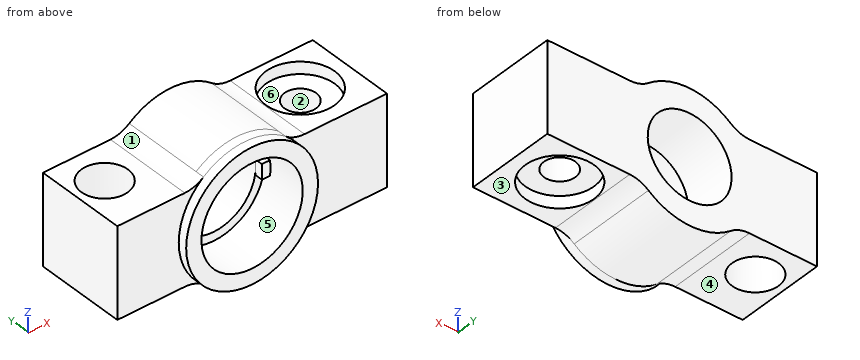
```python
from build123d import *

# Parameters (mm, degrees)
BOSS_EXTRUDE2_DEPTH  = 3
SKETCH3_W            = 20
SKETCH3_H            = 30
BOSS_EXTRUDE5_DEPTH  = 26
SKETCH8_R            = 7.75
CUT_EXTRUDE2_DEPTH   = 36
BOSS_EXTRUDE7_DEPTH  = 27
SKETCH14_R           = 22
BOSS_EXTRUDE8_DEPTH  = 20
SKETCH16_R           = 11.5
CUT_EXTRUDE3_DEPTH   = 4
SKETCH17_R           = 5.25
CUT_EXTRUDE4_DEPTH   = 44
CUT_EXTRUDE5_START   = -4
SKETCH18_R           = 11.5
CUT_EXTRUDE5_DEPTH   = 4
SKETCH24_W           = 6.849841191
SKETCH24_H           = 4
BOSS_EXTRUDE12_DEPTH = 13
SKETCH26_W           = 5
SKETCH26_H           = 30
CUT_EXTRUDE10_DEPTH  = 6
SKETCH27_R           = 22
BOSS_EXTRUDE15_DEPTH = 7
BOSS_EXTRUDE17_DEPTH = 27
SKETCH37_W           = 20
SKETCH37_H           = 30
BOSS_EXTRUDE18_DEPTH = 1
FILLET17_R           = 10
BOSS_EXTRUDE19_START = 3
SKETCH41_R           = 22
BOSS_EXTRUDE19_DEPTH = 3
SKETCH44_W           = 5.842947404
SKETCH44_H           = 4
BOSS_EXTRUDE21_DEPTH = 22
SKETCH46_R           = 16.9
CUT_EXTRUDE11_DEPTH  = 15.5
SKETCH48_R           = 14
CUT_EXTRUDE13_DEPTH  = 25.5
SKETCH49_W           = 5.321549717
SKETCH49_H           = 5
BOSS_EXTRUDE24_DEPTH = 20


with BuildPart() as part:
    # Sketch1 → Boss-Extrude2 (new body)
    with BuildSketch(Plane(origin=(0, 0, 0), x_dir=(1, 0, 0), z_dir=(0, 1, 0))):
        with BuildLine():
            Line((16.093476939, 15), (47.5, 15))
            Line((47.5, 15), (47.5, -15))
            Line((47.5, -15), (16.093476939, -15))
            ThreePointArc((16.093476939, -15), (0, -22), (-16.093476939, -15))
            Line((-16.093476939, -15), (-47.5, -15))
            Line((-47.5, -15), (-47.5, 15))
            Line((-47.5, 15), (-16.093476939, 15))
            ThreePointArc((-16.093476939, 15), (0, 22), (16.093476939, 15))
        make_face()
    extrude(amount=BOSS_EXTRUDE2_DEPTH)

    # Sketch3 → Boss-Extrude5 (add)
    with BuildSketch(Plane(origin=(0, 3, 0), x_dir=(1, 0, 0), z_dir=(0, 1, 0))):
        with Locations((-32.5, 0)):
            Rectangle(SKETCH3_W, SKETCH3_H)
    extrude(amount=BOSS_EXTRUDE5_DEPTH)

    # Sketch8 → Cut-Extrude2 (cut)
    with BuildSketch(Plane.XY.offset(15)):
        with Locations((-32.5, 17.2)):
            Circle(SKETCH8_R)
    extrude(amount=-CUT_EXTRUDE2_DEPTH, mode=Mode.SUBTRACT)

    # Sketch9 → Boss-Extrude7 (add)
    with BuildSketch(Plane(origin=(0, 3, 0), x_dir=(1, 0, 0), z_dir=(0, 1, 0))):
        with BuildLine():
            Line((16.093476939, 15), (47.5, 15))
            Line((47.5, 15), (47.5, -15))
            Line((47.5, -15), (16.093476939, -15))
            ThreePointArc((16.093476939, -15), (22, 0), (16.093476939, 15))
        make_face()
    extrude(amount=BOSS_EXTRUDE7_DEPTH)

    # Sketch14 → Boss-Extrude8 (add)
    with BuildSketch(Plane(origin=(0, 3, 0), x_dir=(1, 0, 0), z_dir=(0, 1, 0))):
        Circle(SKETCH14_R)
    extrude(amount=BOSS_EXTRUDE8_DEPTH)

    # Sketch16 → Cut-Extrude3 (cut)
    with BuildSketch(Plane.XY.offset(15)):
        with Locations((31.79673847, 16)):
            Circle(SKETCH16_R)
    extrude(amount=-CUT_EXTRUDE3_DEPTH, mode=Mode.SUBTRACT)

    # Sketch17 → Cut-Extrude4 (cut)
    with BuildSketch(Plane.XY.offset(11)):
        with Locations((31.79673847, 16)):
            Circle(SKETCH17_R)
    extrude(amount=-CUT_EXTRUDE4_DEPTH, mode=Mode.SUBTRACT)

    # Sketch18 → Cut-Extrude5 (cut)
    with BuildSketch(Plane(origin=(0, 0, -15), x_dir=(-1, 0, 0), z_dir=(0, 0, -1)).offset(CUT_EXTRUDE5_START)):
        with Locations(Location((-31.79673847, 16, 0), (0, 0, 180))):
            Circle(SKETCH18_R)
    extrude(amount=CUT_EXTRUDE5_DEPTH, mode=Mode.SUBTRACT)

    # Sketch24 → Boss-Extrude12 (add)
    with BuildSketch(Plane(origin=(0, 23, 0), x_dir=(1, 0, 0), z_dir=(0, 1, 0))):
        with Locations((17.924920596, 0)):
            Rectangle(SKETCH24_W, SKETCH24_H)
    extrude(amount=-BOSS_EXTRUDE12_DEPTH)

    # Sketch26 → Cut-Extrude10 (cut)
    with BuildSketch(Plane(origin=(0, 3, 0), x_dir=(1, 0, 0), z_dir=(0, 1, 0))):
        with Locations((-45, 0)):
            Rectangle(SKETCH26_W, SKETCH26_H)
    extrude(amount=-CUT_EXTRUDE10_DEPTH, mode=Mode.SUBTRACT)

    # Sketch27 → Boss-Extrude15 (add)
    with BuildSketch(Plane(origin=(0, 23, 0), x_dir=(1, 0, 0), z_dir=(0, 1, 0))):
        Circle(SKETCH27_R)
    extrude(amount=BOSS_EXTRUDE15_DEPTH)

    # Sketch36 → Boss-Extrude17 (add)
    with BuildSketch(Plane(origin=(0, 3, 0), x_dir=(1, 0, 0), z_dir=(0, 1, 0))):
        with BuildLine():
            Line((-16.093476939, -15), (-22.5, -15))
            Line((-22.5, -15), (-22.5, 15))
            Line((-22.5, 15), (-16.093476939, 15))
            ThreePointArc((-16.093476939, 15), (-22, 0), (-16.093476939, -15))
        make_face()
    extrude(amount=BOSS_EXTRUDE17_DEPTH)

    # Sketch37 → Boss-Extrude18 (add)
    with BuildSketch(Plane(origin=(0, 29, 0), x_dir=(1, 0, 0), z_dir=(0, 1, 0))):
        with Locations((-32.5, 0)):
            Rectangle(SKETCH37_W, SKETCH37_H)
    extrude(amount=BOSS_EXTRUDE18_DEPTH)

    # Fillet17
    # the kernel refuses this fillet: 10 mm, written as the material it adds along each edge
    with BuildSketch(Plane(origin=(16.093476939, 3, 15), x_dir=(-0.7334988970942886, 0, 0.67969064136669), z_dir=(0, 1, 0))) as fillet17_piece_1:
        with BuildLine():
            CenterArc((3.949825005, 9.973213236), FILLET17_R, 227.180526604, 38.624832873)
            Line((-2.847081409, 2.638224265), (0, 0))
            ThreePointArc((0, 0), (1.609187965, 0.058930881), (3.21837593, 0))
        make_face()
    extrude(amount=20)
    with BuildSketch(Plane(origin=(-16.093476939, 3, 15), x_dir=(-1, 0, 0), z_dir=(0, 1, 0)), Plane(origin=(16.093476939, 3, -15), x_dir=(1, 0, 0), z_dir=(0, 1, 0))) as fillet17_piece_2:
        with BuildLine():
            CenterArc((3.881507416, 10), FILLET17_R, 231.375167127, 38.624832873)
            ThreePointArc((-2.360675195, 2.1875), (-1.140282829, 1.136975736), (0, 0))
            Line((0, 0), (3.881507416, 0))
        make_face()
    extrude(amount=20)
    with BuildSketch(Plane(origin=(-16.093476939, 3, -15), x_dir=(-1, 0, 0), z_dir=(0, 1, 0))) as fillet17_piece_3:
        with BuildLine():
            CenterArc((3.881507416, -10), FILLET17_R, 90, 38.624832873)
            ThreePointArc((-2.360675195, -2.1875), (-1.140282829, -1.136975736), (0, 0))
            Line((0, 0), (3.881507416, 0))
        make_face()
    extrude(amount=20)
    with BuildSketch(Plane(origin=(16.093476939, 0, -15), x_dir=(1, 0, 0), z_dir=(0, 1, 0)), Plane(origin=(-16.093476939, 0, 15), x_dir=(-1, 0, 0), z_dir=(0, 1, 0))) as fillet17_piece_4:
        with BuildLine():
            CenterArc((3.881507416, 10), FILLET17_R, 231.375167127, 38.624832873)
            ThreePointArc((-2.360675195, 2.1875), (-1.140282829, 1.136975736), (0, 0))
            Line((0, 0), (3.881507416, 0))
        make_face()
    extrude(amount=3)
    with BuildSketch(Plane(origin=(16.093476939, 23, -15), x_dir=(1, 0, 0), z_dir=(0, 1, 0)), Plane(origin=(-16.093476939, 23, 15), x_dir=(-1, 0, 0), z_dir=(0, 1, 0))) as fillet17_piece_5:
        with BuildLine():
            CenterArc((3.881507416, 10), FILLET17_R, 231.375167127, 38.624832873)
            ThreePointArc((-2.360675195, 2.1875), (-1.140282829, 1.136975736), (0, 0))
            Line((0, 0), (3.881507416, 0))
        make_face()
    extrude(amount=7)
    with BuildSketch(Plane(origin=(-16.093476939, 0, -15), x_dir=(0.7334988970942858, 0, -0.6796906413666929), z_dir=(0, 1, 0)), Plane(origin=(16.093476939, 0, 15), x_dir=(-0.7334988970942886, 0, 0.6796906413666898), z_dir=(0, 1, 0))) as fillet17_piece_6:
        with BuildLine():
            CenterArc((3.949825005, 9.973213236), FILLET17_R, 227.180526604, 38.624832873)
            Line((-2.847081409, 2.638224265), (0, 0))
            ThreePointArc((0, 0), (1.609187965, 0.058930881), (3.21837593, 0))
        make_face()
    extrude(amount=3)
    with BuildSketch(Plane(origin=(-16.093476939, 23, -15), x_dir=(-1, 0, 0), z_dir=(0, 1, 0))) as fillet17_piece_7:
        with BuildLine():
            CenterArc((3.881507416, -10), FILLET17_R, 90, 38.624832873)
            ThreePointArc((-2.360675195, -2.1875), (-1.140282829, -1.136975736), (0, 0))
            Line((0, 0), (3.881507416, 0))
        make_face()
    extrude(amount=7)
    with BuildSketch(Plane(origin=(16.093476939, 23, 15), x_dir=(-0.7334988970942886, 0, 0.67969064136669), z_dir=(0, 1, 0))) as fillet17_piece_8:
        with BuildLine():
            CenterArc((3.949825005, 9.973213236), FILLET17_R, 227.180526604, 38.624832873)
            Line((-2.847081409, 2.638224265), (0, 0))
            ThreePointArc((0, 0), (1.609187965, 0.058930881), (3.21837593, 0))
        make_face()
    extrude(amount=7)

    # Sketch41 → Boss-Extrude19 (add)
    with BuildSketch(Plane.XZ.offset(BOSS_EXTRUDE19_START)):
        with Locations(Location((0, 0, 0), (0, 0, 270))):
            Circle(SKETCH41_R)
    extrude(amount=-BOSS_EXTRUDE19_DEPTH)

    # Sketch44 → Boss-Extrude21 (add)
    with BuildSketch(Plane(origin=(0, 30, 0), x_dir=(1, 0, 0), z_dir=(0, 1, 0))):
        with Locations((16.9, 0)):
            Rectangle(SKETCH44_W, SKETCH44_H)
    extrude(amount=-BOSS_EXTRUDE21_DEPTH)

    # Sketch46 → Cut-Extrude11 (cut)
    with BuildSketch(Plane.XZ.offset(3)):
        with Locations(Location((0, 0, 0), (0, 0, 270))):
            Circle(SKETCH46_R)
    extrude(amount=-CUT_EXTRUDE11_DEPTH, mode=Mode.SUBTRACT)

    # Sketch48 → Cut-Extrude13 (cut)
    with BuildSketch(Plane.XZ.offset(-12.5)):
        with Locations(Location((0, 0, 0), (0, 0, 270))):
            Circle(SKETCH48_R)
    extrude(amount=-CUT_EXTRUDE13_DEPTH, mode=Mode.SUBTRACT)

    # Sketch49 → Boss-Extrude24 (add)
    with BuildSketch(Plane(origin=(0, 30, 0), x_dir=(1, 0, 0), z_dir=(0, 1, 0))):
        with Locations((16.690799244, 0)):
            Rectangle(SKETCH49_W, SKETCH49_H)
    extrude(amount=-BOSS_EXTRUDE24_DEPTH)


solid = part.part
```
Work out the finished part from the listing and answer in its coordinate system (mm). Face numbers are marked on the shaded views. A direction names the side the tool comes from. Give positions to 0.01 mm unless a question says otherwise; leave off trailing zeros. Order: outer loops, then holes, each group sorted by start corner. A loop starts at its lowest first (then second) coordinate and runs counter-clockwise, first axis right, second up. Notation, with made-up numbers: (5, 1) - (48, 1) arc R35 ccw to (48, 37) - close; hole circle Ø8 at (49.25, 64.25). An arc over 180 degrees is marked (long way). One line per item, written item: value. Start each with the question number.
1. Which of the six approach directions +Z, -Z, +X, -X, +Y, -Y give full straight-line access (tool end or side, diameter ignored) to the marked faces 4, 5 and 6?
2. Section B-B, the plane x = -32.5 is taken. Write down the section's boundary in (y, z), then the cut area to 3 significant figures.
3. Section D-D, the plane y = 26.5 is taken. Write down the section's boundary in (x, z), then the cut area to 3 significant figures.
4. For a pull along X with two mould halves and no side action, classify the marked faces 1, 2 and 3 as released by +X, released by -X, zero draft, split by the parting line, or undercut.
5. Consider line 1 (Z direction, x = 0, y = 9); line 2 (Y direction, x = -32.5, z = 7.75); line 3 (Y direction, x = -15, z = 2). Determine where each line is inside the solid, lowest interval first.
6. Each of these flat-tipped pins is pushed along its axis until it touches: pin 1 Ø3 at (x, y) = (13, 6) entering from +Z (3 decimals); pin 2 Ø3 at (x, y) = (16, 11.5) entering from -Z; pin 3 Ø11.5 at (x, y) = (-37, 16.5) entering from -Z; pin 4 Ø22.5 at (x, z) = (0, 0) entering from +Y. Where does it stop, or does it pass through?
7. Section A-A, the plane z = 0 is taken. Count the separate pieces of the cut face and the enclosed holes in it, then the cut area to 3 significant figures.
Filled sheet:
1. face 4: -Z, -X, +Y, -Y
1. face 5: -Y
1. face 6: +Z
2. outline: (0, -15) - (9.45, -15) - (9.45, 15) - (0, 15) - close; (24.95, -15) - (30, -15) - (30, 15) - (24.95, 15) - close
2. area: 435 mm²
3. outline: (-42.5, -15) - (-19.97, -15) arc R10 cw to (-13.73, -17.19) arc R22 ccw to (13.73, -17.19) arc R10 cw to (19.97, -15) - (27.11, -15) - (27.11, -11) - (36.49, -11) - (36.49, -15) - (47.5, -15) - (47.5, 15) - (36.49, 15) - (36.49, 11) - (27.11, 11) - (27.11, 15) - (19.97, 15) arc R10 cw to (13.73, 17.19) arc R22 ccw to (-13.73, 17.19) arc R10 cw to (-19.97, 15) - (-42.5, 15) - close; hole circle Ø28 at (0, 0)
3. area: 2,330 mm²
4. face 1: released by -X
4. face 2: undercut
4. face 3: zero draft
5. line 1: -22 to -16.9, 16.9 to 22
5. line 2: 0 to 9.45, 24.95 to 30
5. line 3: 12.5 to 30
6. pin 1: z = 18.755
6. pin 2: z = -16.63
6. pin 3: z = -15
6. pin 4: through
7. separate pieces: 2
7. enclosed holes: 2
7. area: 1,550 mm²
